For this review, use the dimensioned drawing (mm, ordinates from the lowest corner) and the shaded views. Give positions to 0.01 mm unless a question says otherwise; leave off trailing zeros. Write each loop counter-clockwise with the first axis right and the second up, starting at its lowest first coordinate (ties: lowest second). Pieces come first, ordered by that corner, then holes. Notation, with made-up numbers: M -17.5,71.25 L 6.5,71.25 A26 ccw 6.5,107.25 Z; hole C 31.5,-17 d8. An arc over 180 degrees is marked long. One line per item, written item: value. Start each with the question number.
Item 1: To check wall thickness, follow probe 1 along Y at (x, z) = (4.7, 151.5); probe 2 along Z at (x, y) = (1.7, 4.75). State the ranges of each line that lie inside material, in increasing order.
Item 2: Clearance check with a flat-ended pin moving along its axis: pin 1 Ø1.8 at (x, z) = (4, 8) entering from -Y. State where the tip first meets the part, or that it passes through.
Item 3: Consider section B-B, the plane x = 1.2. Write out the cut boundary in (y, z).
Item 4: Consider section C-C, the plane z = 171. Write out the cut boundary in (x, y), and give its area (3 significant figures).
Item 5: Consider section A-A, the plane y = 3.5. Write out the cut boundary in (x, z).
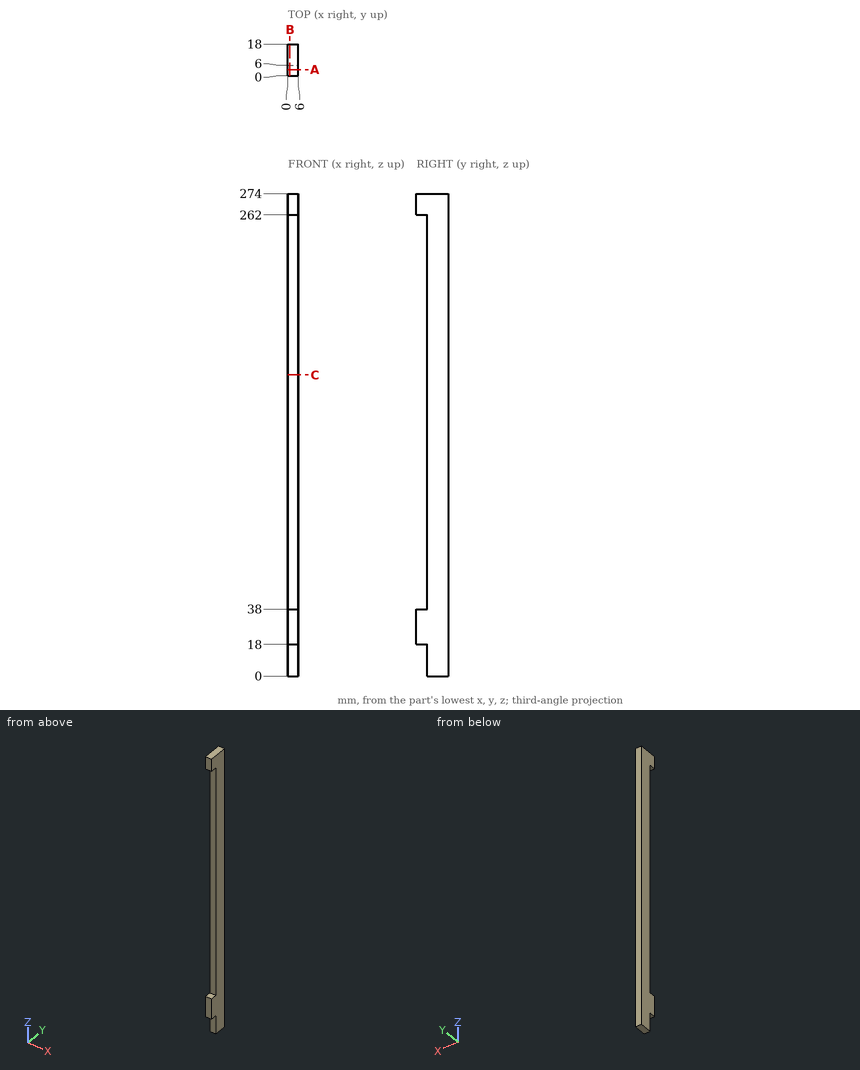
Model answer:
1. probe 1: y = 6 to 18
1. probe 2: z = 18 to 38, 262 to 274
2. pin 1: stops at y = 6
3. outline: M 0,18 L 6,18 L 6,0 L 18,0 L 18,274 L 0,274 L 0,262 L 6,262 L 6,38 L 0,38 Z
4. outline: M 0,6 L 6,6 L 6,18 L 0,18 Z
4. area: 72.0 mm2
5. outline: M 0,18 L 6,18 L 6,38 L 0,38 Z; M 0,262 L 6,262 L 6,274 L 0,274 Z
